Build history of the part. All positions in model axes, mm. Face numbers are marked on the shaded views. A direction names the side the tool comes from. Coordinates: 2 decimals unless noted, no trailing zeros. Loops run counter-clockwise (first coordinate to the right, second up) from the corner with the lowest first, then second, coordinate; pieces in that order, holes last.
(1) Slice it at C-C (y = 15.5). Give the cut face in (x, z), and give its area (3 significant figures).
(2) Wall check: L1, parallel to X at y = 23, z = -48.5; L2, parallel to Z at x = -13.5, y = 24; L3, parallel to Y at x = 19, z = 8.5. Give the ranges that are in metal, low to high.
(3) Slice it at B-B (x = -1.5). Give the cut face in (y, z).
(4) Tool access for the marked faces 1, 2, 3, 4 and 5: list every direction of +Z, -Z, +X, -X, +Y, -Y with a clear straight run to the whole face (end or side of a thin tool).
(5) Flat gauge pins, fed straight in: P1, Ø10, axis at x = 6.5, y = 8.5, coming from the +Z side; P2, Ø8, axis at y = 7.5, z = 43, coming from the +X side; P3, Ø1.1, axis at x = 5.5, y = 12.5, coming from the +Z side. Where does each tip first touch, or does it go through?
(6) Slice it at A-A (z = -13). Give the cut face in (x, y), and give its area (3 significant figures).
(7) Slice it at D-D (y = 5.5). Give the cut face in (x, z), and give its area (3 significant figures).
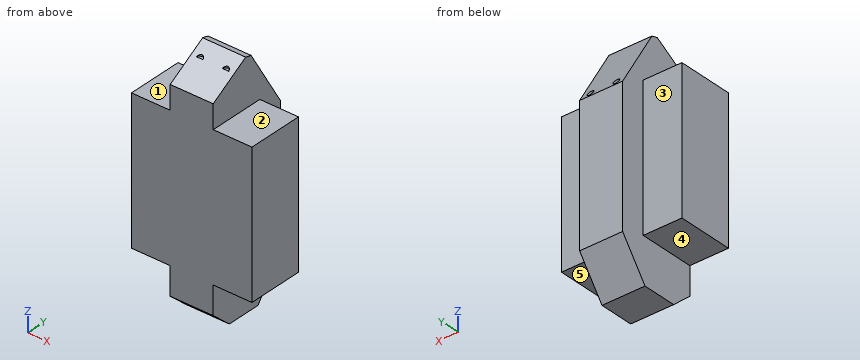
from build123d import *

# Parameters (mm, degrees)
SKETCH_1_W           = 20
SKETCH_1_H           = 110
EXTRUDE_1_DEPTH      = 38
EXTRUDE_4_DEPTH      = 32
EXTRUDE_4_DEPTH_BACK = 34
SKETCH_2_W           = 18
SKETCH_2_H           = 26
CUT_EXTRUDE_1_DEPTH  = 20
SKETCH_9_R           = 1.5
CUT_EXTRUDE_3_DEPTH  = 5
SKETCH_10_W          = 99.275483207
SKETCH_10_H          = 3
CUT_EXTRUDE_4_DEPTH  = 77.896033708
SKETCH_8_R           = 1.5
CUT_EXTRUDE_2_DEPTH  = 5
CUT_EXTRUDE_5_DEPTH  = 77.650179387
CUT_EXTRUDE_6_DEPTH  = 77.650179387
CHAMFER_1_SIZE       = 2.2


with BuildPart() as part:
    # 草图1 → 凸台-拉伸1 (new body)
    with BuildSketch(Plane(origin=(0, 0, 0), x_dir=(1, 0, 0), z_dir=(0, 1, 0))):
        Rectangle(SKETCH_1_W, SKETCH_1_H)
    extrude(amount=EXTRUDE_1_DEPTH)

    # 草图2 → 凸台-拉伸4 (add, two sides: drawn at the far end of the back side and taken through both)
    with BuildSketch(Plane.XY.offset(-EXTRUDE_4_DEPTH_BACK)):
        with Locations((19, 13)):
            Rectangle(SKETCH_2_W, SKETCH_2_H)
        with Locations((-19, 13)):
            Rectangle(SKETCH_2_W, SKETCH_2_H)
    extrude(amount=EXTRUDE_4_DEPTH + EXTRUDE_4_DEPTH_BACK)

    # 草图7 → 切除-拉伸1 (cut)
    with BuildSketch(Plane(origin=(10, 0, 0), x_dir=(0, 0, -1), z_dir=(1, 0, 0))):
        Polygon((-55, 38), (-55, 20), (-25.042969318, 38), align=None)
    extrude(amount=-CUT_EXTRUDE_1_DEPTH, mode=Mode.SUBTRACT)

    # 草图9 → 切除-拉伸3 (cut)
    with BuildSketch(Plane.XY.offset(55)):
        with Locations((-6, 11.5)):
            Circle(SKETCH_9_R)
        with Locations(Location((6, 11.5, 0), (0, 0, 180))):
            Circle(SKETCH_9_R)
    extrude(amount=-CUT_EXTRUDE_3_DEPTH, mode=Mode.SUBTRACT)

    # 草图10 → 切除-拉伸4 (cut, through all)
    with BuildSketch(Plane(origin=(10, 0, 0), x_dir=(0, 0, -1), z_dir=(1, 0, 0))):
        with Locations((8.83578939, 39)):
            Rectangle(SKETCH_10_W, SKETCH_10_H)
    extrude(amount=-CUT_EXTRUDE_4_DEPTH, mode=Mode.SUBTRACT)

    # 草图8 → 切除-拉伸2 (cut)
    with BuildSketch(Plane(origin=(0, 38.975774431, 23.419007952), x_dir=(1, 0, 0), z_dir=(0, 0.8571673007021134, 0.5150380749100524))):
        with Locations(Location((-6, -5.305369578, 0), (0, 0, 270))):
            Circle(SKETCH_8_R)
        with Locations(Location((6, -5.305369578, 0), (0, 0, 90))):
            Circle(SKETCH_8_R)
    extrude(amount=-CUT_EXTRUDE_2_DEPTH, mode=Mode.SUBTRACT)

    # 草图11 → 切除-拉伸5 (cut, through all)
    with BuildSketch(Plane(origin=(10, 0, 0), x_dir=(0, 0, -1), z_dir=(1, 0, 0))):
        Polygon((55, 37.5), (38, 37.5), (55, 25), align=None)
        Polygon((55, 0), (55, 9), (47, 0), align=None)
    extrude(amount=-CUT_EXTRUDE_5_DEPTH, mode=Mode.SUBTRACT)

    # 草图12 → 切除-拉伸6 (cut, through all)
    with BuildSketch(Plane(origin=(10, 0, 0), x_dir=(0, 0, -1), z_dir=(1, 0, 0))):
        Polygon((-55, 20), (-42.982787619, 0), (-55, 0), align=None)
    extrude(amount=-CUT_EXTRUDE_6_DEPTH, mode=Mode.SUBTRACT)

    # 倒角1
    chamfer_1_edges = [part.edges().sort_by_distance(p)[0] for p in [
        (0, 20, 55),
    ]]
    chamfer(chamfer_1_edges, length=CHAMFER_1_SIZE)


solid = part.part
Response values:
1. outline: (-28, -34) - (-10, -34) - (-10, -55) - (10, -55) - (10, -34) - (28, -34) - (28, 32) - (10, 32) - (10, 52.3) - (-10, 52.3) - (-10, 32) - (-28, 32) - close
1. area: 4,520 mm2
2. L1: x = -10 to 10
2. L2: z = -34 to 32
2. L3: y = 0 to 26
3. outline: (0, -47) - (9, -55) - (25, -55) - (37.5, -38) - (37.5, 25.88) - (21.13, 53.11) - (18.11, 53.87) - (0, 42.98) - close
4. face 1: +Z, -X, +Y, -Y
4. face 2: +Z, +X, +Y, -Y
4. face 3: +Z, -Z, -X, +Y
4. face 4: -Z, -X, +Y, -Y
4. face 5: -Z, +X, +Y, -Y
5. P1: stops at z = 51.09
5. P2: stops at x = 10
5. P3: stops at z = 50.82
6. outline: (-28, 0) - (28, 0) - (28, 26) - (10, 26) - (10, 37.5) - (-10, 37.5) - (-10, 26) - (-28, 26) - close
6. area: 1,690 mm2
7. outline: (-28, -34) - (-10, -34) - (-10, -51.89) - (10, -51.89) - (10, -34) - (28, -34) - (28, 32) - (10, 32) - (10, 46.29) - (-10, 46.29) - (-10, 32) - (-28, 32) - close
7. area: 4,340 mm2
